```python
from build123d import *

# Parameters (mm, degrees)
SKETCH1_R           = 4.15925
SKETCH1_R_2         = 2.4511
BOSS_EXTRUDE1_DEPTH = 10.287
SKETCH2_OUTSIDE_W   = 13.444
SKETCH2_OUTSIDE_H   = 13.444
SKETCH2_OUTSIDE_R   = 2.97815
CUT_EXTRUDE1_DEPTH  = 6.731
CHAMFER1_SIZE       = 1.778
CHAMFER1_SIZE2      = 1.339819101


with BuildPart() as part:
    # Sketch1 → Boss-Extrude1 (new body)
    with BuildSketch(Plane.XY):
        Circle(SKETCH1_R)
        Circle(SKETCH1_R_2, mode=Mode.SUBTRACT)
    extrude(amount=BOSS_EXTRUDE1_DEPTH)

    # Sketch2 outside → Cut-Extrude1 (cut)
    with BuildSketch(Plane.XY.offset(10.287)):
        Rectangle(SKETCH2_OUTSIDE_W, SKETCH2_OUTSIDE_H)
        Circle(SKETCH2_OUTSIDE_R, mode=Mode.SUBTRACT)
    extrude(amount=-CUT_EXTRUDE1_DEPTH, mode=Mode.SUBTRACT)

    # Chamfer1
    chamfer1_edges = [part.edges().sort_by_distance(p)[0] for p in [
        (-2.4511, 0, 0),
    ]]
    chamfer1_side = [part.faces().sort_by_distance(p)[0] for p in [
        (-2.4511, 0, 5.1435),
    ]]
    chamfer(chamfer1_edges, length=CHAMFER1_SIZE, length2=CHAMFER1_SIZE2, reference=chamfer1_side[0])


solid = part.part
```
The model under review builds one solid part; all positions refer to its coordinate system, in mm. Round coordinates to 2 decimals unless told otherwise and drop trailing zeros. Order: outer loops, then holes, each group sorted by start corner. A loop starts at its lowest first (then second) coordinate and runs counter-clockwise, first axis right, second up. Notation, with made-up numbers: (2, 21) -> (6, 21) arc R9 cw to (6, 36) -> close; hole circle Ø10 at (-40, 70.25). An arc over 180 degrees is marked (long way). One line per item, written item: value. Start each with the question number.
Q1. Clearance check with a flat-ended pin moving along its axis: pin 1 Ø4 at (x, z) = (-2.5, 3) entering from -Y. State where the tip first meets the part, or that it passes through.
Q2. Wall thickness on line 1 (Y direction, x = 0, z = 7.75); line 2 (Y direction, x = 1.25, z = 3); line 3 (Z direction, x = -0.5, y = 4): over which ranges is each line inside the solid? List them lowest first.
Q3. Mouldability with a two-part tool opening along X and no side actions: class faces 1 (the face through (-2.363, -1.812, 6.969)), 2 (the face through (-3, 1, 3.556)), 3 (the face through (2.338, 0.736, 5.973)) as released by +X, released by -X, zero draft, split by the parting line, or undercut.
Q4. Take a section at A-A (x = 0). Write out the cut boundary in (y, z).
Q5. Take a section at C-C (z = 6.5). Write out the cut boundary in (x, y), and give its area (3 significant figures).
Reported:
1. pin 1: stops at y = -4.13
2. line 1: y = -2.98 to -2.45, 2.45 to 2.98
2. line 2: y = -3.97 to -2.11, 2.11 to 3.97
2. line 3: z = 0 to 3.56
3. face 1: split by the parting line
3. face 2: zero draft
3. face 3: undercut
4. outline: (-4.16, 0) -> (-3.79, 0) -> (-2.45, 1.78) -> (-2.45, 10.29) -> (-2.98, 10.29) -> (-2.98, 3.56) -> (-4.16, 3.56) -> close; (2.45, 1.78) -> (3.79, 0) -> (4.16, 0) -> (4.16, 3.56) -> (2.98, 3.56) -> (2.98, 10.29) -> (2.45, 10.29) -> close
5. outline: circle Ø5.96 at (0, 0); hole circle Ø4.9 at (0, 0)
5. area: 8.99 mm2
